from build123d import *

# Parameters (mm, degrees)
F0_W     = 1524
F0_H     = 254
F1_DEPTH = 25.4
F2_R     = 25.4
F3_DEPTH = 12.7


with BuildPart() as f1:
    # F0 (on Top) → F1 (new body, symmetric)
    with BuildSketch(Plane.XY):
        with Locations((631.803309, 98.702285)):
            Rectangle(F0_W, F0_H)
    extrude(amount=F1_DEPTH, both=True)

    # F2 (on face) → F3 (cut)
    with BuildSketch(Plane.XY.offset(25.4)):
        with Locations((-66.696691, 98.702285)):
            Circle(F2_R)
    extrude(amount=-F3_DEPTH, mode=Mode.SUBTRACT)


solid = f1.part
Source: CAD feature listing. Evaluate the final solid. Frame: model axes, mm. A direction names the side the tool comes from. Round coordinates to 2 decimals unless told otherwise and drop trailing zeros. Use a Markdown table: item, result. Add a question column.
1. Set-up query: faces 1 (the cylindrical face through (-92.072, 99.819, 19.139)), 2 (the flat face through (1393.803, 97, 0)). Return all of +Z, -Z, +X, -X, +Y, -Y with unobstructed straight access to the full face (end or side cutting, diameter ignored); none if empty.
2. Mould query, pull axis Y, two halves, no side actions, for faces 3 (the flat face through (621, -28.298, 0)), 4 (the flat face through (-67, 99, 12.7)), 5 (the flat face through (621, 225.702, 0)), 6 (the flat face through (621, 100, 25.4)). Classes: +Y half, -Y half, draft (parallel to the pull), parting line (faces both ways), or undercut.
3. First-contact query: pin 1 (15 mm diameter, centred on x = -62, y = 90.5, fed in from +Z). Flat tip, straight axial feed; report the tip coordinate or a pass-through.
Derived:
| question | item | result |
|---|---|---|
| 1 | face 1 | +Z |
| 1 | face 2 | +Z, -Z, +X, +Y, -Y |
| 2 | face 3 | -Y half |
| 2 | face 4 | undercut |
| 2 | face 5 | +Y half |
| 2 | face 6 | draft |
| 3 | pin 1 | z = 12.7 |
